Job drawing, mm, ordinate dimensions from the low corner. One solid piece. A direction names the side the tool comes from. Give positions to 0.01 mm unless a question says otherwise; leave off trailing zeros. Loops run counter-clockwise (first coordinate to the right, second up) from the corner with the lowest first, then second, coordinate; pieces in that order, holes last. Notation, with made-up numbers: M 14.5,-29.75 L 56.5,-29.75 A16 cw 56.5,-18.75 Z; hole C -31.5,57 d7. An arc over 180 degrees is marked long. Answer as CSV lines item,"result".
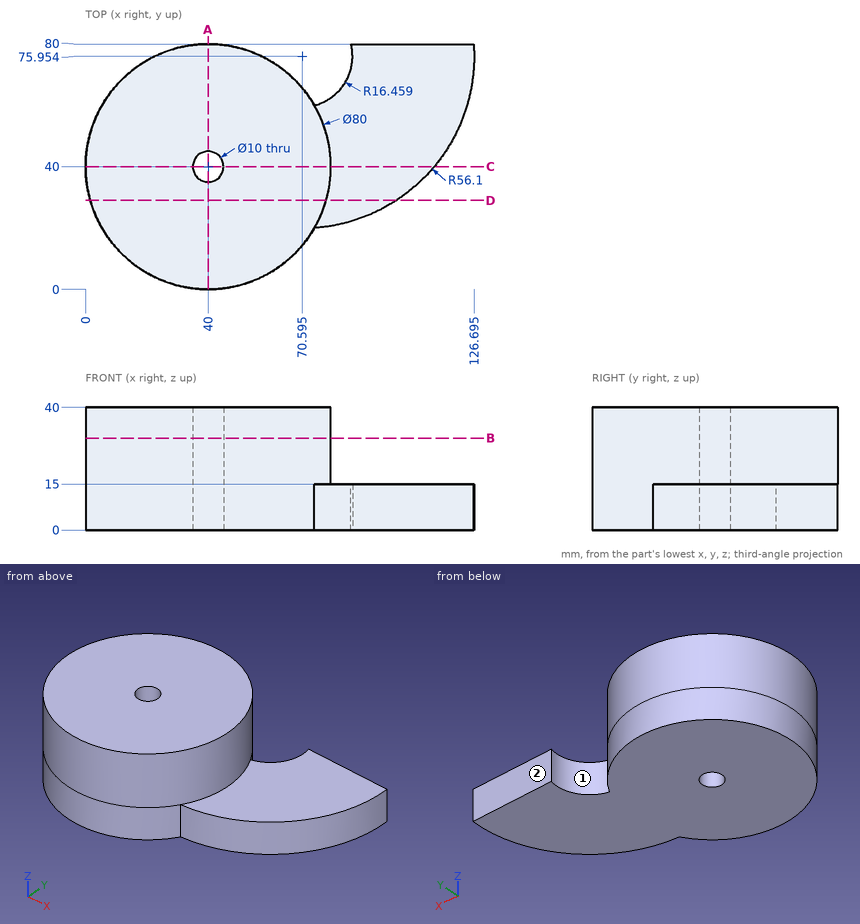
1) Flat gauge pins, fed straight in: pin 1 (12 mm diameter, centred on x = 53.5, z = 34.5, fed in from +Y); pin 2 (10 mm diameter, centred on x = 24.5, z = 15, fed in from +Y); pin 3 (8 mm diameter, centred on y = 57.5, z = 35, fed in from -X). Where does each tip first touch, or does it go through?
Answer below:
pin 1,"stops at y = 79.29"
pin 2,"stops at y = 78.6"
pin 3,"stops at x = 2.35"
2) Drill centre lines: line 1 (Y direction, x = 40, z = 32.5); line 2 (Z direction, x = 97.5, y = 62.5); line 3 (X direction, y = 35.5, z = 35) (1 decimal). Where is each one in solid material? Low to high. Write a range as from..to.
Answer below:
line 1,"y = 0..35, 45..80"
line 2,"z = 0..15"
line 3,"x = 0.3..37.8, 42.2..79.7"
3) Band-saw the part on A-A on x = 40. Give the cut face in (y, z).
Answer below:
outline,"M 0,0 L 35,0 L 35,40 L 0,40 Z; M 45,0 L 80,0 L 80,40 L 45,40 Z"
4) Band-saw the part on C-C on y = 40. Give the cut face in (x, z), and give its area (4 significant figures).
Answer below:
outline,"M 0,0 L 35,0 L 35,40 L 0,40 Z; M 45,0 L 113.66,0 L 113.66,15 L 80,15 L 80,40 L 45,40 Z"
area,"3,305 mm^2"
5) Band-saw the part on B-B on z = 30. Give the cut face in (x, y), and give its area (3 significant figures).
Answer below:
outline,"C 40,40 d80; hole C 40,40 d10"
area,"4,950 mm^2"
6) Which spindle directions (+Z, -Z, +X, -X, +Y, -Y) get a long thin tool onto all of the face, cutting with end or side? Do the marked faces 1 and 2. Say none if no direction does.
Answer below:
face 1,"+Z, -Z"
face 2,"+Z, -Z, +X, -X, +Y"
7) Band-saw the part on D-D on y = 29. Give the cut face in (x, z).
Answer below:
outline,"M 1.54,0 L 101.3,0 L 101.3,15 L 78.46,15 L 78.46,40 L 1.54,40 Z"
